Autodesk Inventor part; units mm, degrees
ref_plane "YZ Plane" through (0, 0, 0) normal (1, 0, 0) x (0, 1, 0)
ref_plane "XZ Plane" through (0, 0, 0) normal (0, 1, 0) x (-1, 0, 0)
ref_plane "XY Plane" through (0, 0, 0) normal (0, 0, 1) x (1, 0, 0)
sketch "Sketch1" plane through (0, 0, 0) normal (0, 0, 1) x (1, 0, 0)
  line L0 (-37, 65.25) -> (37, 65.25)
  line L1 (-37, 53.25) -> (37, 53.25)
  line L2 (35, 65.25) -> (35, 53.25)
  line L3 (7.056, 209) -> (7.056, 197)
  line L4 (7.056, 209) -> (7.056, 197)
  line L5 (9.056, 197) -> (7.056, 197)
  line L6 (7.056, 209) -> (11.056, 209)
  line L7 (35, 53.25) -> (39, 53.25)
  line L8 (39, 53.25) -> (39, 57.25)
  line L9 (39, 57.25) -> (37, 57.25)
  line L10 (37, 57.25) -> (37, 61.25)
  line L11 (37, 61.25) -> (39, 61.25)
  line L12 (39, 61.25) -> (39, 65.25)
  line L13 (39, 65.25) -> (37, 65.25) construction
  line L14 (11.056, 209) -> (11.056, 205)
  line L15 (11.056, 205) -> (9.056, 205)
  line L16 (9.056, 205) -> (9.056, 201)
  line L17 (9.056, 201) -> (11.056, 201)
  line L18 (11.056, 201) -> (11.056, 197)
  line L19 (39, 65.25) -> (47.9764, 69.6572)
  line L20 (37, 65.25) -> (45.9764, 69.6572)
  line L21 (37, 65.25) -> (37, 83.6946) construction
  line L22 (45.9764, 69.6572) -> (37, 69.6572) construction
  line L23 (45.9764, 69.6572) -> (37, 74.0645)
  line L24 (47.9764, 69.6572) -> (39, 74.0645)
  line L25 (35.5321, 190.0108) -> (11.056, 197.3225)
  line L26 (37, 188.6524) -> (9.056, 197)
  line L27 (37, 74.0645) -> (46.1526, 74.0645) construction
  line L28 (45.9764, 78.4717) -> (37, 82.8789)
  line L29 (47.9764, 78.4717) -> (39, 82.8789)
  line L30 (39, 74.0645) -> (47.9764, 78.4717)
  line L31 (37, 74.0645) -> (45.9764, 78.4717)
  line L32 (45.9764, 87.2861) -> (37, 91.6934)
  line L33 (47.9764, 87.2861) -> (39, 91.6934)
  line L34 (39, 82.8789) -> (47.9764, 87.2861)
  line L35 (37, 82.8789) -> (45.9764, 87.2861)
  line L36 (45.9764, 96.1006) -> (37, 100.5078)
  line L37 (47.9764, 96.1006) -> (39, 100.5078)
  line L38 (39, 91.6934) -> (47.9764, 96.1006)
  line L39 (37, 91.6934) -> (45.9764, 96.1006)
  line L40 (45.9764, 104.915) -> (37, 109.3223)
  line L41 (47.9764, 104.915) -> (39, 109.3223)
  line L42 (39, 100.5078) -> (47.9764, 104.915)
  line L43 (37, 100.5078) -> (45.9764, 104.915)
  line L44 (45.9764, 113.7295) -> (37, 118.1367)
  line L45 (47.9764, 113.7295) -> (39, 118.1367)
  line L46 (39, 109.3223) -> (47.9764, 113.7295)
  line L47 (37, 109.3223) -> (45.9764, 113.7295)
  line L48 (45.9764, 122.5439) -> (37, 126.9512)
  line L49 (47.9764, 122.5439) -> (39, 126.9512)
  line L50 (39, 118.1367) -> (47.9764, 122.5439)
  line L51 (37, 118.1367) -> (45.9764, 122.5439)
  line L52 (45.9764, 131.3584) -> (37, 135.7656)
  line L53 (47.9764, 131.3584) -> (39, 135.7656)
  line L54 (39, 126.9512) -> (47.9764, 131.3584)
  line L55 (37, 126.9512) -> (45.9764, 131.3584)
  line L56 (45.9764, 140.1729) -> (37, 144.5801)
  line L57 (47.9764, 140.1729) -> (39, 144.5801)
  line L58 (39, 135.7656) -> (47.9764, 140.1729)
  line L59 (37, 135.7656) -> (45.9764, 140.1729)
  line L60 (45.9764, 148.9873) -> (37, 153.3945)
  line L61 (47.9764, 148.9873) -> (39, 153.3945)
  line L62 (39, 144.5801) -> (47.9764, 148.9873)
  line L63 (37, 144.5801) -> (45.9764, 148.9873)
  line L64 (45.9764, 157.8018) -> (37, 162.209)
  line L65 (47.9764, 157.8018) -> (39, 162.209)
  line L66 (39, 153.3945) -> (47.9764, 157.8018)
  line L67 (37, 153.3945) -> (45.9764, 157.8018)
  line L68 (45.9764, 166.6162) -> (37, 171.0234)
  line L69 (47.9764, 166.6162) -> (39, 171.0234)
  line L70 (39, 162.209) -> (47.9764, 166.6162)
  line L71 (37, 162.209) -> (45.9764, 166.6162)
  line L72 (45.9764, 175.4307) -> (37, 179.8379)
  line L73 (47.9764, 175.4307) -> (39, 179.8379)
  line L74 (39, 171.0234) -> (47.9764, 175.4307)
  line L75 (37, 171.0234) -> (45.9764, 175.4307)
  line L76 (0, -41.8) -> (0, 250.8)
  line L77 (-9, 209) -> (9, 209) construction
  line L78 (45.9764, 184.2451) -> (37, 188.6524)
  line L79 (47.9764, 184.2451) -> (39, 188.6524)
  line L80 (39, 179.8379) -> (47.9764, 184.2451)
  line L81 (37, 179.8379) -> (45.9764, 184.2451)
  arc A0 (39, 188.6524) -> (35.5321, 190.0108) centre (29.1072, 168.5031) ccw
  point P0 (0, 0)
  point P1 (37, 195.25)
  dimension "d0" = 4
  dimension "d1" = 12
  dimension "d2" = 4
  dimension "d3" = 2
  dimension "d4" = 2
  dimension "d5" = 4
  dimension "d6" = 4
  dimension "d7" = 2
  dimension "d8" = 2
  dimension "d12" = 116.15
  dimension "d13" = 0.8814
  dimension "d17" = 10
  dimension "d18" = 8.8145
  dimension "d28" = 8.8145
  dimension "d34" = 12
  dimension "d35" = 4
  dimension "RevolveDIA" = 7.056
  dimension "d39" = 106.632
  dimension "d40" = 2
  dimension "d41" = 0.8814
revolve "Revolution1" add sketch "Sketch1" angle 360 about axis through (0, -10, 0) along (0, 1, 0) contours L0 L20 L23 L31 L28 L35 L32 L39 L36 L43 L40 L47 L44 L51 L48 L55 L52 L59 L56 L63 L60 L67 L64 L71 L68 L75 L72 L81 L78 L26 L5 L3 L6 L14 L15 L16 L17 L18 L25 A0 L79 L80 L73 L74 L69 L70 L65 L66 L61 L62 L57 L58 L53 L54 L49 L50 L45 L46 L41 L42 L37 L38 L33 L34 L29 L30 L24 L19 L12 L11 L10 L9 L8 L7 L1 L2
equation "\"d0\" = 0.333333 * d1"
equation "\"d2\" = d0"
equation "\"d5\" = d0"
equation "\"d6\" = d0"
equation "\"d28\" = d18"
equation "\"d40\" = d7"
equation "\"d41\" = d13"
equation "\"d10\" = d9"
properties part number "MCEN4000:T7" material "RUBBER, SILICONE"
CAD build for the part. Positions are in the model's coordinates, mm. A direction names the side the tool comes from. Round coordinates to 2 decimals unless told otherwise and drop trailing zeros. Order: outer loops, then holes, each group sorted by start corner. A loop starts at its lowest first (then second) coordinate and runs counter-clockwise, first axis right, second up. Notation, with made-up numbers: (-12.75, 69.25) - (6.25, 69.25) arc R16 ccw to (6.25, 98.25) - close; hole circle Ø11 at (-15, -32). An arc over 180 degrees is marked (long way). Use CSV: the item, a comma, the result in double quotes. Start each with the question number.
1) Tool access for faces 3 (the conical face through (-4.89, 91.42, 37.24)), 4 (the cylindrical face through (-1.44, 199.14, 10.96)): list every direction of +Z, -Z, +X, -X, +Y, -Y with a clear straight run to the whole face (end or side of a thin tool).
2) Saw through at A-A (y = 63.5). List the corners of the cut face in (x, z), and give its area (3 significant figures).
3) Wall check: L1, parallel to X at y = 58.75, z = 0; L2, parallel to X at y = 204, z = 0; L3, parallel to Z at x = 0, y = 206. Give the ranges that are in metal, low to high. Write a range as [from, to].
4) Pin check, flat tips, straight feed: pin 1 Ø6 at (y, z) = (169, -3.5) entering from +X; pin 2 Ø2 at (x, z) = (20.5, 34.5) entering from +Y; pin 3 Ø22 at (x, z) = (-18.5, 5) entering from +Y; pin 4 Ø20 at (x, z) = (3, -1.5) entering from -Y. Stop position of each tip, or through.
5) Two-plate mould, pull along Y, no slides. Class faces 1 (the conical face through (35.83, 171.3, -11.28)), 2 (the cylindrical face through (-5.077, 55.278, -38.668)): pulls with the +Y half, pulls with the -Y half, needs draft (parallel to the pull), parting line crosses it, or undercut.
Values follow:
1,face 3,"none"
1,face 4,"+Y"
2,outline,"circle Ø78 at (0, 0); hole circle Ø70 at (0, 0)"
2,area,"930 mm2"
3,L1,"x = [-37, -35], [35, 37]"
3,L2,"x = [-9.06, -7.06], [7.06, 9.06]"
3,L3,"z = [-11.06, -7.06], [7.06, 11.06]"
4,pin 1,"stops at x = 47.95"
4,pin 2,"stops at y = 188.59"
4,pin 3,"stops at y = 209"
4,pin 4,"stops at y = 195.72"
5,face 1,"undercut"
5,face 2,"needs draft"
